Drawing for the job (mm, zero at the part's lowest x, y, z). Coordinates: 2 decimals unless noted, no trailing zeros. Order: outer loops, then holes, each group sorted by start corner. A loop starts at its lowest first (then second) coordinate and runs counter-clockwise, first axis right, second up. Notation, with made-up numbers: (88, 64.25) -> (122, 64.25) arc R13 cw to (122, 77.25) -> close; hole circle Ø7 at (36.5, 39). An arc over 180 degrees is marked (long way). Write each question's results on one line, items separated by ' | '.
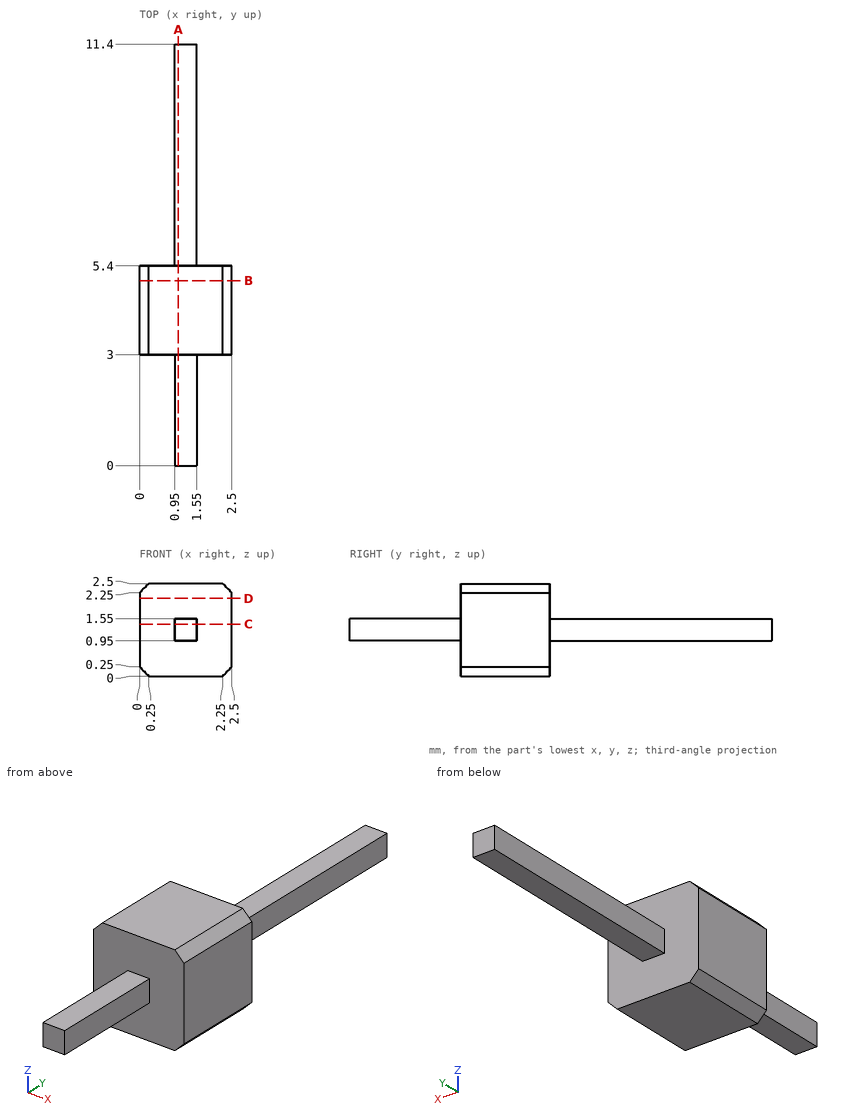
Item 1: Slice it at A-A, the plane x = 1.05. List the corners of the cut face in (y, z).
Answer:
outline: (0, 0.95) -> (3, 0.95) -> (3, 0) -> (5.4, 0) -> (5.4, 0.95) -> (11.4, 0.95) -> (11.4, 1.55) -> (5.4, 1.55) -> (5.4, 2.5) -> (3, 2.5) -> (3, 1.55) -> (0, 1.55) -> close
Item 2: Slice it at C-C, the plane z = 1.4. List the corners of the cut face in (x, y), and give its area (3 significant figures).
Answer:
outline: (0, 3) -> (0.95, 3) -> (0.95, 0) -> (1.55, 0) -> (1.55, 3) -> (2.5, 3) -> (2.5, 5.4) -> (1.55, 5.4) -> (1.55, 11.4) -> (0.95, 11.4) -> (0.95, 5.4) -> (0, 5.4) -> close | area: 11.4 mm^2
Item 3: Slice it at B-B, the plane y = 5. List the corners of the cut face in (x, z), and give its area (4 significant figures).
Answer:
outline: (0, 0.25) -> (0.25, 0) -> (2.25, 0) -> (2.5, 0.25) -> (2.5, 2.25) -> (2.25, 2.5) -> (0.25, 2.5) -> (0, 2.25) -> close | area: 6.125 mm^2
Item 4: Pin check, flat tips, straight feed: pin 1 (0.7 mm diameter, centred on x = 1, y = 7.5, fed in from +Z); pin 2 (0.5 mm diameter, centred on y = 1.5, z = 1.5, fed in from +X); pin 3 (0.7 mm diameter, centred on x = 1, y = 1.5, fed in from -Z). Stop position of each tip, or through.
Answer:
pin 1: stops at z = 1.55 | pin 2: stops at x = 1.55 | pin 3: stops at z = 0.95
Item 5: Slice it at D-D, the plane z = 2.1. List the corners of the cut face in (x, y).
Answer:
outline: (0, 3) -> (2.5, 3) -> (2.5, 5.4) -> (0, 5.4) -> close
Item 6: Drill centre lines: line 1 (Y direction, x = 1.1, z = 0.55); line 2 (Z direction, x = 1.4, y = 1). Where is each one in solid material? Low to high. Write a range as from..to.
Answer:
line 1: y = 3..5.4 | line 2: z = 0.95..1.55
